Could you check a few things on this model? Use its own coordinates, in mm. A direction names the side the tool comes from. Give positions to 0.01 mm unless a question says otherwise; leave off trailing zeros. Write each loop counter-clockwise with the first axis right and the second up, starting at its lowest first coordinate (ties: lowest second). Pieces come first, ordered by that corner, then holes. Notation, with made-up numbers: M 9.25,-15 L 13.25,-15 A14 cw 13.25,3 Z; hole C -25.5,-6 d1. An arc over 180 degrees is marked long. Use one line per item in the form item = value.
from build123d import *

# Parameters (mm, degrees)
SKICA1_W                 = 50
SKICA1_H                 = 50
P_IDAT_VYSUNUT_M2_DEPTH  = 3
SKICA5_W                 = 5
SKICA5_H                 = 22.5
ODEBRAT_VYSUNUT_M3_DEPTH = 1
P_IDAT_VYSUNUT_M9_DEPTH  = 15
SKICA17_R                = 2
ODEBRAT_VYSUNUT_M8_DEPTH = 4
ZAOBLIT1_R               = 10
ZAOBLIT2_R               = 5


with BuildPart() as part:
    # Skica1 → Přidat vysunutím2 (new body)
    with BuildSketch(Plane.XY):
        Rectangle(SKICA1_W, SKICA1_H)
    extrude(amount=P_IDAT_VYSUNUT_M2_DEPTH)

    # Skica5 → Odebrat vysunutím3 (cut)
    with BuildSketch(Plane(origin=(0, 0, 0), x_dir=(-1, 0, 0), z_dir=(0, 0, -1))):
        Polygon((-25, -2.5), (-2.5, -2.5), (2.5, -2.5), (2.5, 2.5), (-25, 2.5), align=None)
        with Locations((0, -13.75)):
            Rectangle(SKICA5_W, SKICA5_H)
    extrude(amount=-ODEBRAT_VYSUNUT_M3_DEPTH, mode=Mode.SUBTRACT)

    # Skica14 → Přidat vysunutím9 (add)
    with BuildSketch(Plane.XY.offset(3)):
        Polygon((25, 25), (-25, 25), (-25, -25), (-24, -25), (-24, 24), (24, 24), (24, -25), (25, -25), align=None)
    extrude(amount=P_IDAT_VYSUNUT_M9_DEPTH)

    # Skica17 → Odebrat vysunutím8 (cut)
    with BuildSketch(Plane(origin=(0, 0, 1), x_dir=(-1, 0, 0), z_dir=(0, 0, -1))):
        with Locations((-16, 0)):
            Circle(SKICA17_R)
        with Locations((0, -16)):
            Circle(SKICA17_R)
    extrude(amount=-ODEBRAT_VYSUNUT_M8_DEPTH, mode=Mode.SUBTRACT)

    # Zaoblit1
    zaoblit1_edges = [part.edges().sort_by_distance(p)[0] for p in [
        (-2.5, 2.5, 0.5),
    ]]
    fillet(zaoblit1_edges, radius=ZAOBLIT1_R)

    # Zaoblit2
    zaoblit2_edges = [part.edges().sort_by_distance(p)[0] for p in [
        (2.5, -2.5, 0.5),
    ]]
    fillet(zaoblit2_edges, radius=ZAOBLIT2_R)


solid = part.part
1) For faces 1 (the flat face through (0, 25, 9)), 2 (the flat face through (24, 0, 10)), 3 (the cylindrical face through (0.51, -0.35, 0.51)), which set-ups out of +Z, -Z, +X, -X, +Y, -Y let a thin tool reach every point of the face, with its end or its side?
Checked values:
face_1 = +Z, -Z, +X, -X, +Y
face_2 = +Z, -Y
face_3 = -Z
2) Thinking about a two-plate mould opening in X: for faces 4 (the flat face through (8, -2, 1)), 5 (the cylindrical face through (4, -3.93, 0.51)), 6 (the flat face through (25, 0, 9)), 7 (the flat face through (14, -14, 0)), which applies, released by +X, released by -X, zero draft, split by the parting line, or undercut?
Checked values:
face_4 = undercut
face_5 = undercut
face_6 = released by +X
face_7 = zero draft
3) I want a section at A-A, the plane x = 16. Please give me the cut outline in (y, z).
Checked values:
outline = M -25,0 L -2.5,0 L -2.5,1 L -2,1 L -2,3 L -25,3 Z; M 2,1 L 2.5,1 L 2.5,0 L 25,0 L 25,18 L 24,18 L 24,3 L 2,3 Z
4) For pin 1 Ø24 at (x, y) = (6.5, 10.5) entering from +Z; pin 2 Ø3 at (x, z) = (-6, 12.5) entering from -Y, each with a flat end and sliding along its axis, tell me the tip position at first contact or that it passes through.
Checked values:
pin_1 = 3
pin_2 = 24
5) I want a section at C-C, the plane y = 4.5. Please give me the cut outline in (x, z).
Checked values:
outline = M -25,0 L 25,0 L 25,18 L 24,18 L 24,3 L -24,3 L -24,18 L -25,18 Z
6) If I drill on L1, parallel to X at y = -1, z = 15.25; L2, parallel to Y at x = 16, z = 2.25; L3, parallel to Y at x = 0, z = 1.5, over which ranges is the centre line in solid material (lowest first)?
Checked values:
L1 = -25 to -24, 24 to 25
L2 = -25 to -2, 2 to 25
L3 = -25 to -18, -14 to 25
7) I want a section at D-D, the plane x = -13.5. Please give me the cut outline in (y, z), plus the area to 3 significant figures.
Checked values:
outline = M -25,0 L 25,0 L 25,18 L 24,18 L 24,3 L -25,3 Z
area = 165 mm2
8) I want a section at B-B, the plane y = -16. Please give me the cut outline in (x, z), plus the area to 3 significant figures.
Checked values:
outline = M -25,0 L -2.5,0 L -2.5,1 L -2,1 L -2,3 L -24,3 L -24,18 L -25,18 Z; M 2,1 L 2.5,1 L 2.5,0 L 25,0 L 25,18 L 24,18 L 24,3 L 2,3 Z
area = 167 mm2
